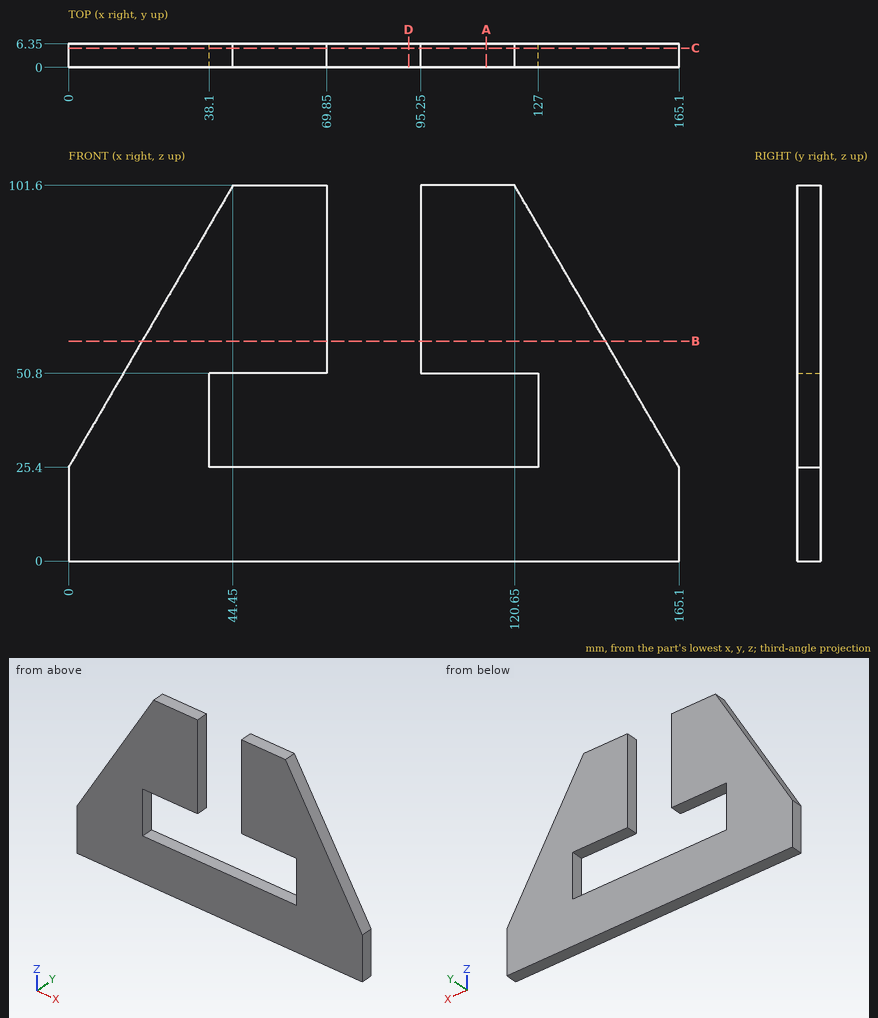
Source: three-view drawing plus pictorial views. Frame: mm from the lowest corner of the part. Round coordinates to 2 decimals unless told otherwise and drop trailing zeros. Order: outer loops, then holes, each group sorted by start corner. A loop starts at its lowest first (then second) coordinate and runs counter-clockwise, first axis right, second up. Notation, with made-up numbers: (60.5, 4) -> (93.5, 4) arc R26 cw to (93.5, 23) -> close; hole circle Ø2 at (76.25, 58.5). An arc over 180 degrees is marked (long way). Use one line per item in the form item = value. Start each with the question number.
1. Cut plane C-C (y = 5.25). Return the cut outline in (x, z).
2. Pin query (flat end, axial travel): pin 1 Ø1.9 at (y, z) = (3.5, 75.5) entering from +X; pin 2 Ø3 at (y, z) = (3.5, 28.5) entering from -X; pin 3 Ø1.9 at (y, z) = (4.5, 35.5) entering from -X; pin 4 Ø8 at (x, z) = (147, 48.5) entering from -Y. Return the tip coordinate at first contact, or that it passes through.
3. Cut plane D-D (x = 92). Return the cut outline in (y, z), then the cut area to 3 significant figures.
4. Cut plane A-A (x = 113). Return the cut outline in (y, z), then the cut area to 3 significant figures.
5. Cut plane B-B (z = 59.5). Return the cut outline in (x, y).
6. Line query: probe 1 along Z at (x, y) = (67, 5.5); probe 2 along Z at (x, y) = (86, 3); probe 3 along X at (y, z) = (5.75, 45.5) (3 decimals). Output: solid intervals per line, ascending.
Solution:
q1.outline = (0, 0) -> (165.1, 0) -> (165.1, 25.4) -> (120.65, 101.6) -> (95.25, 101.6) -> (95.25, 50.8) -> (127, 50.8) -> (127, 25.4) -> (38.1, 25.4) -> (38.1, 50.8) -> (69.85, 50.8) -> (69.85, 101.6) -> (44.45, 101.6) -> (0, 25.4) -> close
q2.pin_1 = 136.43
q2.pin_2 = 0.93
q2.pin_3 = 5.34
q2.pin_4 = 0
q3.outline = (0, 0) -> (6.35, 0) -> (6.35, 25.4) -> (0, 25.4) -> close
q3.area = 161 mm^2
q4.outline = (0, 0) -> (6.35, 0) -> (6.35, 25.4) -> (0, 25.4) -> close; (0, 50.8) -> (6.35, 50.8) -> (6.35, 101.6) -> (0, 101.6) -> close
q4.area = 484 mm^2
q5.outline = (19.89, 0) -> (69.85, 0) -> (69.85, 6.35) -> (19.89, 6.35) -> close; (95.25, 0) -> (145.21, 0) -> (145.21, 6.35) -> (95.25, 6.35) -> close
q6.probe_1 = 0 to 25.4, 50.8 to 101.6
q6.probe_2 = 0 to 25.4
q6.probe_3 = 11.725 to 38.1, 127 to 153.375
